from build123d import *

# Parameters (mm, degrees)
F0_W     = 22.225
F0_H     = 12.7
F0_R     = 2.38125
F1_DEPTH = 9.525
F2_R     = 1.35255
F3_DEPTH = 9.525
F4_W     = 9.525
F4_H     = 3.175
F5_DEPTH = 9.525


with BuildPart() as f1:
    # F0 (on Top) → F1 (new body)
    with BuildSketch(Plane.XY):
        with Locations((11.1125, 6.35)):
            Rectangle(F0_W, F0_H)
        with Locations((11.1125, 4.7625)):
            Circle(F0_R, mode=Mode.SUBTRACT)
    extrude(amount=F1_DEPTH)

    # F2 (on face) → F3 (cut)
    with BuildSketch(Plane(origin=(0, 12.7, 0), x_dir=(-1, 0, 0), z_dir=(0, 1, 0))):
        with Locations((-3.175, 4.7625)):
            Circle(F2_R)
        with Locations((-19.05, 4.7625)):
            Circle(F2_R)
    extrude(amount=-F3_DEPTH, mode=Mode.SUBTRACT)

    # F4 (on face) → F5 (cut, through all)
    with BuildSketch(Plane(origin=(0, 0, 0), x_dir=(1, 0, 0), z_dir=(0, 0, -1))):
        with Locations((11.1125, -11.1125)):
            Rectangle(F4_W, F4_H)
    extrude(amount=-F5_DEPTH, mode=Mode.SUBTRACT)


solid = f1.part
Source: CAD feature listing. Evaluate the final solid. Frame: model axes, mm. A direction names the side the tool comes from. Round coordinates to 2 decimals unless told otherwise and drop trailing zeros. Loops run counter-clockwise (first coordinate to the right, second up) from the corner with the lowest first, then second, coordinate; pieces in that order, holes last. Notation, with made-up numbers: (34.5, 74) - (80.5, 74) arc R14 cw to (80.5, 99) - close; hole circle Ø1 at (-32, 66.25). An arc over 180 degrees is marked (long way). Write item = value, one per line. Start each with the question number.
(1) Section query B-B, the plane x = 12.5. Output: boundary loops of the cut face in (y, z) (3 decimals).
(2) Pull-direction query (Z, two-part tool) for faces 1 (the face through (6.35, 11, 5)), 2 (the face through (11, 8, 9.525)), 3 (the face through (3, 3.175, 5)), 4 (the face through (17.76, 8, 5.17)); classes: +Z half, -Z half, draft (parallel to the pull), parting line (faces both ways), or undercut.
(3) Section query A-A, the plane y = 6.75. State how many separate pieces and enclosed holes the cut face has, plus the area to 3 significant figures.
(4) Ray query, line 1 along X through (y, z) = (10.25, 2.5) (3 decimals); line 2 along X through (y, z) = (11.5, 4) (3 decimals); line 3 along Z through (x, y) = (19.05, 7.75) (3 decimals). Return the intervals inside material, ascending. Write a range as from..to.
(5) Pin query (flat end, axial travel): pin 1 (2.5 mm diameter, centred on x = 19.05, z = 4.76, fed in from +Y) (3 decimals); pin 2 (1 mm diameter, centred on x = 11, z = 3, fed in from +Y) (3 decimals). Return the tip coordinate at first contact, or that it passes through.
(6) Set-up query: faces 5 (the face through (15.875, 11, 5)), 6 (the face through (0, 6, 5)), 7 (the face through (4.526, 8.004, 4.822)). Return all of +Z, -Z, +X, -X, +Y, -Y with unobstructed straight access to the full face (end or side cutting, diameter ignored); none if empty.
(7) Section query D-D, the plane x = 19.05. Output: boundary loops of the cut face in (y, z) (3 decimals).
Conclusion:
q1.outline = (0, 0) - (2.827, 0) - (2.827, 9.525) - (0, 9.525) - close; (6.698, 0) - (9.525, 0) - (9.525, 9.525) - (6.698, 9.525) - close
q2.face_1 = draft
q2.face_2 = +Z half
q2.face_3 = undercut
q2.face_4 = undercut
q3.separate_pieces = 2
q3.enclosed_holes = 2
q3.area = 175 mm2
q4.line_1 = 0..6.35, 15.875..22.225
q4.line_2 = 0..2.058, 4.292..6.35, 15.875..17.933, 20.167..22.225
q4.line_3 = 0..3.41, 6.115..9.525
q5.pin_1 = 3.175
q5.pin_2 = 9.525
q6.face_5 = +Z, -Z, +Y
q6.face_6 = +Z, -Z, -X, +Y, -Y
q6.face_7 = +Y
q7.outline = (0, 0) - (12.7, 0) - (12.7, 3.41) - (3.175, 3.41) - (3.175, 6.115) - (12.7, 6.115) - (12.7, 9.525) - (0, 9.525) - close
